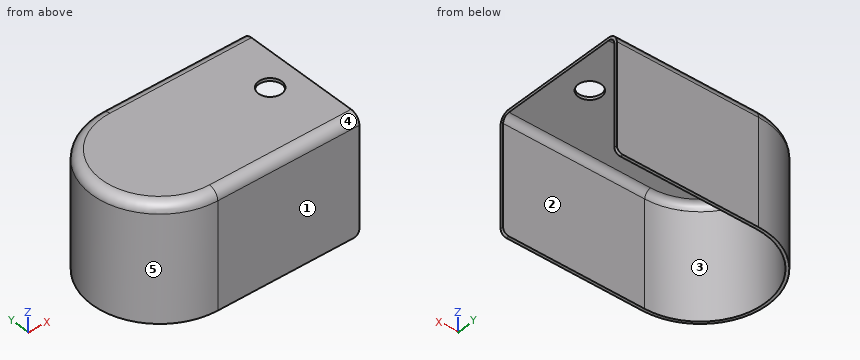
Solid Edge part; units mm, degrees
sketch "Sketch1" plane through (0, 0, 0) normal (0, 0, 1) x (1, 0, 0)
  line L0 (-16.4125, 59.7004) -> (57.0875, 59.7004)
  line L1 (57.0875, 59.7004) -> (57.0875, -10.2996)
  line L2 (57.0875, -10.2996) -> (-16.4125, -10.2996)
  arc A0 (-16.4125, -10.2996) -> (-16.4125, 59.7004) centre (-16.4125, 24.7004) cw
extrude "Protrusion1" add sketch "Sketch1" along normal blind 60
fillet "Round_1" radius 5 3 edges at (-51.4125, 24.7004, 60) (20.3375, 59.7004, 60) (20.3375, -10.2996, 60)
shell "Thinwall_1" thickness 1.5 removed faces 2 at (57.0875, 48.7337, 49.4) at (40.0892, 2.0671, 0)
sketch "Sketch2" plane through (4.5875, 24.7004, 58.5) normal (0, 0, -1) x (-1, 0, 0)
  circle A0 centre (-37.4274, 1.2277) radius 6
extrude "Cutout1" cut sketch "Sketch2" against normal through all
fillet "Round_2" radius 3 2 edges at (57.0875, -9.5496, 0) (57.0875, 58.9504, 0)
Model file for the job. Use its own axes, mm. Face numbers are marked on the shaded views. A direction names the side the tool comes from. Round coordinates to 2 decimals unless told otherwise and drop trailing zeros. Write each loop counter-clockwise with the first axis right and the second up, starting at its lowest first coordinate (ties: lowest second). Pieces come first, ordered by that corner, then holes. Notation, with made-up numbers: (88.5, -27) - (98.5, -27) arc R25 ccw to (98.5, 2) - close; hole circle Ø10 at (24.5, -20). An arc over 180 degrees is marked (long way). Use CSV: the item, a comma, the result in double quotes. Start each with the question number.
Item 1: Pin check, flat tips, straight feed: P1, Ø4, axis at x = -28.5, z = 14, coming from the -Y side; P2, Ø1.5, axis at y = 23.5, z = 18, coming from the +X side; P3, Ø5, axis at x = 2, y = 5, coming from the -Z side. Stop position of each tip, or through.
Item 2: Band-saw the part on A-A (z = 47.5). Write the cut outline in (x, y).
Item 3: Band-saw the part on B-B (x = 18). Write the cut outline in (y, z), and give its area (3 significant figures).
Item 4: Drill centre lines: L1, parallel to Y at x = 42.5, z = 30; L2, parallel to Z at x = -1, y = 33.5; L3, parallel to Y at x = -26, z = 19. Where is each one in solid material? Low to high. Write a range as [from, to].
Item 5: Two-plate mould, pull along Y, no slides. Class the marked faces 3, 4 and 5: released by +Y, released by -Y, zero draft, split by the parting line, or undercut.
Item 6: Tool access for the marked faces 1 and 2: list every direction of +Z, -Z, +X, -X, +Y, -Y with a clear straight run to the whole face (end or side of a thin tool).
Checked values:
1,P1,"stops at y = -8.81"
1,P2,"stops at x = -49.86"
1,P3,"stops at z = 58.5"
2,outline,"(-16.41, -10.3) - (57.09, -10.3) - (57.09, -8.8) - (-16.41, -8.8) arc R33.5 cw to (-16.41, 58.2) - (57.09, 58.2) - (57.09, 59.7) - (-16.41, 59.7) arc R35 ccw to start"
3,outline,"(-10.3, 0) - (-8.8, 0) - (-8.8, 55) arc R3.5 cw to (-5.3, 58.5) - (54.7, 58.5) arc R3.5 cw to (58.2, 55) - (58.2, 0) - (59.7, 0) - (59.7, 55) arc R5 ccw to (54.7, 60) - (-5.3, 60) arc R5 ccw to (-10.3, 55) - close"
3,area,"275 mm²"
4,L1,"y = [-10.3, -8.8], [58.2, 59.7]"
4,L2,"z = [58.5, 60]"
4,L3,"y = [-8.96, -7.4], [56.8, 58.36]"
5,face 3,"undercut"
5,face 4,"released by -Y"
5,face 5,"split by the parting line"
6,face 1,"+Z, -Z, +X, -X, -Y"
6,face 2,"-Z, +X"
